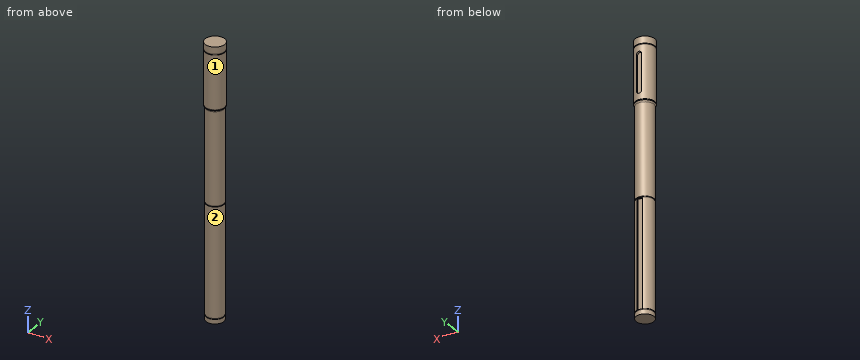
from build123d import *

# Parameters (mm, degrees)
SKETCH2_R           = 10
BOSS_EXTRUDE1_DEPTH = 235
SKETCH3_R           = 10
SKETCH3_R_2         = 9.43
CUT_EXTRUDE2_DEPTH  = 1.1
SKETCH4_W           = 6
SKETCH4_H           = 3.067792635
CUT_EXTRUDE3_DEPTH  = 61.25
SKETCH5_R           = 11
BOSS_EXTRUDE2_DEPTH = 70
FILLET3_R           = 2
SKETCH6_R           = 11
SKETCH6_R_2         = 10.35
CUT_EXTRUDE4_DEPTH  = 1.1
CUT_EXTRUDE5_DEPTH  = 2.5


with BuildPart() as part:
    # Sketch2 → Boss-Extrude1 (new body)
    with BuildSketch(Plane.XY):
        with Locations(Location((0, 0, 0), (0, 0, 180))):
            Circle(SKETCH2_R)
    extrude(amount=BOSS_EXTRUDE1_DEPTH)

    # Sketch3 → Cut-Extrude2 (cut)
    with BuildSketch(Plane(origin=(0, 0, 5), x_dir=(-1, 0, 0), z_dir=(0, 0, -1))):
        Circle(SKETCH3_R)
        Circle(SKETCH3_R_2, mode=Mode.SUBTRACT)
    cut_extrude2 = extrude(amount=-CUT_EXTRUDE2_DEPTH, mode=Mode.SUBTRACT)

    # Mirror1: Cut-Extrude2 across plane
    add(cut_extrude2.mirror(Plane(origin=(0, 0, 67.35), x_dir=(1, 0, 0), z_dir=(0, 0, -1))), mode=Mode.SUBTRACT)

    # Sketch4 → Cut-Extrude3 (cut, symmetric)
    with BuildSketch(Plane(origin=(0, 0, 67.35), x_dir=(-1, 0, 0), z_dir=(0, 0, -1))):
        with Locations((0, 9.343896318)):
            Rectangle(SKETCH4_W, SKETCH4_H)
    extrude(amount=CUT_EXTRUDE3_DEPTH, both=True, mode=Mode.SUBTRACT)

    # Sketch5 → Boss-Extrude2 (add)
    with BuildSketch(Plane.XY.offset(235)):
        Circle(SKETCH5_R)
    extrude(amount=BOSS_EXTRUDE2_DEPTH)

    # Fillet3
    # the kernel refuses this fillet: 2 mm, written as the material it adds along each edge
    with BuildSketch(Plane(origin=(0, 0, 235), x_dir=(-1, 0, 0), z_dir=(0, 1, 0))) as fillet3_piece_1:
        with BuildLine():
            CenterArc((12, -1.732050808), FILLET3_R, 120, 60)
            Line((10, -1.732050808), (9.96, -1.732050808))
            Line((9.96, -1.732050808), (9.96, 0))
            Line((9.96, 0), (10, 0.04))
            ThreePointArc((10, 0.04), (10.5, 0.04), (10.98, 0.034641016))
            Line((10.98, 0.034641016), (11, 0))
        make_face()
    revolve(axis=Axis((0, 0, 235), (0, 0, 1)))

    # Sketch6 → Cut-Extrude4 (cut)
    with BuildSketch(Plane.XY.offset(235)):
        Circle(SKETCH6_R)
        Circle(SKETCH6_R_2, mode=Mode.SUBTRACT)
    cut_extrude4 = extrude(amount=CUT_EXTRUDE4_DEPTH, mode=Mode.SUBTRACT)

    # Mirror2: Cut-Extrude4 across plane
    add(cut_extrude4.mirror(Plane.XY.offset(266.1)), mode=Mode.SUBTRACT)

    # Sketch8 → Cut-Extrude5 (cut)
    with BuildSketch(Plane(origin=(0, 11, 0), x_dir=(1, 0, 0), z_dir=(0, 1, 0))):
        with BuildLine():
            Line((3, -246.1), (3, -286.1))
            ThreePointArc((3, -286.1), (0, -289.1), (-3, -286.1))
            Line((-3, -286.1), (-3, -246.1))
            ThreePointArc((-3, -246.1), (0, -243.1), (3, -246.1))
        make_face()
    extrude(amount=-CUT_EXTRUDE5_DEPTH, mode=Mode.SUBTRACT)


solid = part.part
For this review, take the finished solid that the model builds, in its own axes (mm). Face numbers are marked on the shaded views. A direction names the side the tool comes from. Round coordinates to 2 decimals unless told otherwise and drop trailing zeros. Loops run counter-clockwise (first coordinate to the right, second up) from the corner with the lowest first, then second, coordinate; pieces in that order, holes last. Notation, with made-up numbers: (-23.75, 37) - (0.25, 37) arc R11 cw to (0.25, 48) - close; hole circle Ø5 at (15.5, 33). An arc over 180 degrees is marked (long way). Use one line per item in the form item = value.
Item 1: Consider section B-B on z = 119. Write out the cut boundary in (x, y).
Answers:
outline = (-3, 7.81) - (-3, 9.54) arc R10 ccw (long way) to (3, 9.54) - (3, 7.81) - close
Item 2: Clearance check with flat-ended pins moving along their axes: P1, Ø1.4, axis at y = 8.5, z = 94, coming from the -X side; P2, Ø10, axis at x = -0.5, z = 31, coming from the +Y side; P3, Ø1, axis at x = -8.5, z = 47.5, coming from the -Y side. State where each tip first meets the part, or that it passes through.
Answers:
P1 = -6.26
P2 = 9.54
P3 = -6
Item 3: Tool access review of the marked faces 1 and 2: name each direction out of +Z, -Z, +X, -X, +Y, -Y from which nothing blocks a thin tool from reaching the whole face with its end or side.
Answers:
face_1 = +Z, -Z
face_2 = -Z
Item 4: For line 1 (Z direction, x = -0.5, y = 9.5); line 2 (Z direction, x = -2.5, y = 8.25); line 3 (Z direction, x = -9.75, y = 4.25), list the stretches that pass through material, from the lowest coordinate up.
Answers:
line_1 = 0 to 5, 129.7 to 243.14, 289.06 to 305
line_2 = 0 to 6.1, 128.6 to 305
line_3 = 234.73 to 235, 236.1 to 296.1, 297.2 to 305
Item 5: Consider section A-A on z = 213.5. Write out the cut boundary in (x, y), then the cut area to 3 significant figures.
Answers:
outline = circle Ø20 at (0, 0)
area = 314 mm^2
